Work out the finished part from the listing and answer in its coordinate system (mm). A direction names the side the tool comes from. Give positions to 0.01 mm unless a question says otherwise; leave off trailing zeros. Order: outer loops, then holes, each group sorted by start corner. A loop starts at its lowest first (then second) coordinate and runs counter-clockwise, first axis right, second up.
```python
from build123d import *

# Parameters (mm, degrees)
ESQUISSE1_R             = 9.5
BOSS_EXTRU_1_DEPTH      = 8
CONG_1_R                = 1
CONG_2_R                = 1
CONG_3_R                = 7
ESQUISSE2_R             = 2
ENL_V_MAT_EXTRU_1_DEPTH = 6


with BuildPart() as part:
    # Esquisse1 → Boss.-Extru.1 (new body)
    with BuildSketch(Plane.XY):
        with BuildLine():
            Line((14, -8.053746339), (28, -8.053746339))
            Line((28, -8.053746339), (28, -13.053746339))
            Line((28, -13.053746339), (-28, -13.053746339))
            Line((-28, -13.053746339), (-28, -8.053746339))
            Line((-28, -8.053746339), (-14, -8.053746339))
            Line((-14, -8.053746339), (-14, 0))
            ThreePointArc((-14, 0), (0, 14), (14, 0))
            Line((14, 0), (14, -8.053746339))
        make_face()
        Circle(ESQUISSE1_R, mode=Mode.SUBTRACT)
    extrude(amount=BOSS_EXTRU_1_DEPTH)

    # Congé1
    cong_1_edges = [part.edges().sort_by_distance(p)[0] for p in [
        (-9.5, 0, 8),
    ]]
    fillet(cong_1_edges, radius=CONG_1_R)

    # Congé2
    cong_2_edges = [part.edges().sort_by_distance(p)[0] for p in [
        (-9.5, 0, 0),
    ]]
    fillet(cong_2_edges, radius=CONG_2_R)

    # Congé3
    cong_3_edges = [part.edges().sort_by_distance(p)[0] for p in [
        (-14, -8.053746339, 4),
        (14, -8.053746339, 4),
    ]]
    fillet(cong_3_edges, radius=CONG_3_R)

    # Esquisse2 → Enlèv. mat.-Extru.1 (cut)
    with BuildSketch(Plane(origin=(0, -8.053746339, 0), x_dir=(1, 0, 0), z_dir=(0, 1, 0))):
        with Locations(Location((24.5, -4, 0), (0, 0, 270))):
            Circle(ESQUISSE2_R)
        with Locations(Location((-24.5, -4, 0), (0, 0, 270))):
            Circle(ESQUISSE2_R)
    extrude(amount=-ENL_V_MAT_EXTRU_1_DEPTH, mode=Mode.SUBTRACT)


solid = part.part
```
1. The mould has two halves that part along Z. Classify faces 4 (the face through (-27, -8.054, 4)), 5 (the face through (0, -11, 8)), 6 (the face through (22.548, -10.519, 3.566)): pulls with the +Z half, pulls with the -Z half, needs draft (parallel to the pull), parting line crosses it, or undercut.
Findings below:
face 4: needs draft
face 5: pulls with the +Z half
face 6: undercut
2. The part is cut by section C-C (x = 23.5). Write down the section's boundary in (y, z).
Findings below:
outline: (-13.05, 0) - (-8.05, 0) - (-8.05, 2.27) - (-13.05, 2.27) - close; (-13.05, 5.73) - (-8.05, 5.73) - (-8.05, 8) - (-13.05, 8) - close
3. Given P1, Ø6, axis at x = -6.5, y = 3.5, coming from the -Z side; P2, Ø2, axis at x = 20.5, z = 4.5, coming from the +Y side; P3, Ø1.2, axis at y = -0.5, z = 6, coming from the +X side, each flat-ended and moving along its own axis, determine where each tip first touches the part or whether it passes through.
Findings below:
P1: stops at z = 0.01
P2: stops at y = -7.89
P3: stops at x = 14
4. Which of the six approach directions +Z, -Z, +X, -X, +Y, -Y give full straight-line access (tool end or side, diameter ignored) to faces 1 (the face through (4.38, -8.43, 3.96)), 2 (the face through (-14, -0.5, 3.9)), 3 (the face through (22, -8.054, 4))?
Findings below:
face 1: +Z, -Z
face 2: +Z, -Z, -X, +Y
face 3: +Z, -Z, +X, +Y
5. Straight lines are drawn through the part: probe 1 along X at (y, z) = (-10.4, 4); probe 2 along Y at (x, z) = (0, 3.5); probe 3 along X at (y, z) = (0.25, 3). For each, find the intervals that lie inside material, in ascending order.
Findings below:
probe 1: x = -28 to -26.5, -22.5 to 22.5, 26.5 to 28
probe 2: y = -13.05 to -9.5, 9.5 to 14
probe 3: x = -14 to -9.5, 9.5 to 14
6. The part is cut by section D-D (x = 16.5). Write down the section's boundary in (y, z).
Findings below:
outline: (-13.05, 0) - (-6.42, 0) - (-6.42, 8) - (-13.05, 8) - close
7. The part is cut by section A-A (x = -24.5). Write down the section's boundary in (y, z), then the cut area to 3 significant figures.
Findings below:
outline: (-13.05, 0) - (-8.05, 0) - (-8.05, 2) - (-13.05, 2) - close; (-13.05, 6) - (-8.05, 6) - (-8.05, 8) - (-13.05, 8) - close
area: 20.0 mm2
8. The part is cut by section B-B (z = 4). Write down the section's boundary in (x, y), then the cut area to 3 significant figures.
Findings below:
outline: (-28, -13.05) - (-26.5, -13.05) - (-26.5, -8.05) - (-28, -8.05) - close; (-22.5, -13.05) - (22.5, -13.05) - (22.5, -8.05) - (21, -8.05) arc R7 cw to (14, -1.05) - (14, 0) arc R14 ccw to (-14, 0) - (-14, -1.05) arc R7 cw to (-21, -8.05) - (-22.5, -8.05) - close; (26.5, -13.05) - (28, -13.05) - (28, -8.05) - (26.5, -8.05) - close; hole circle Ø19 at (0, 0)
area: 511 mm2
